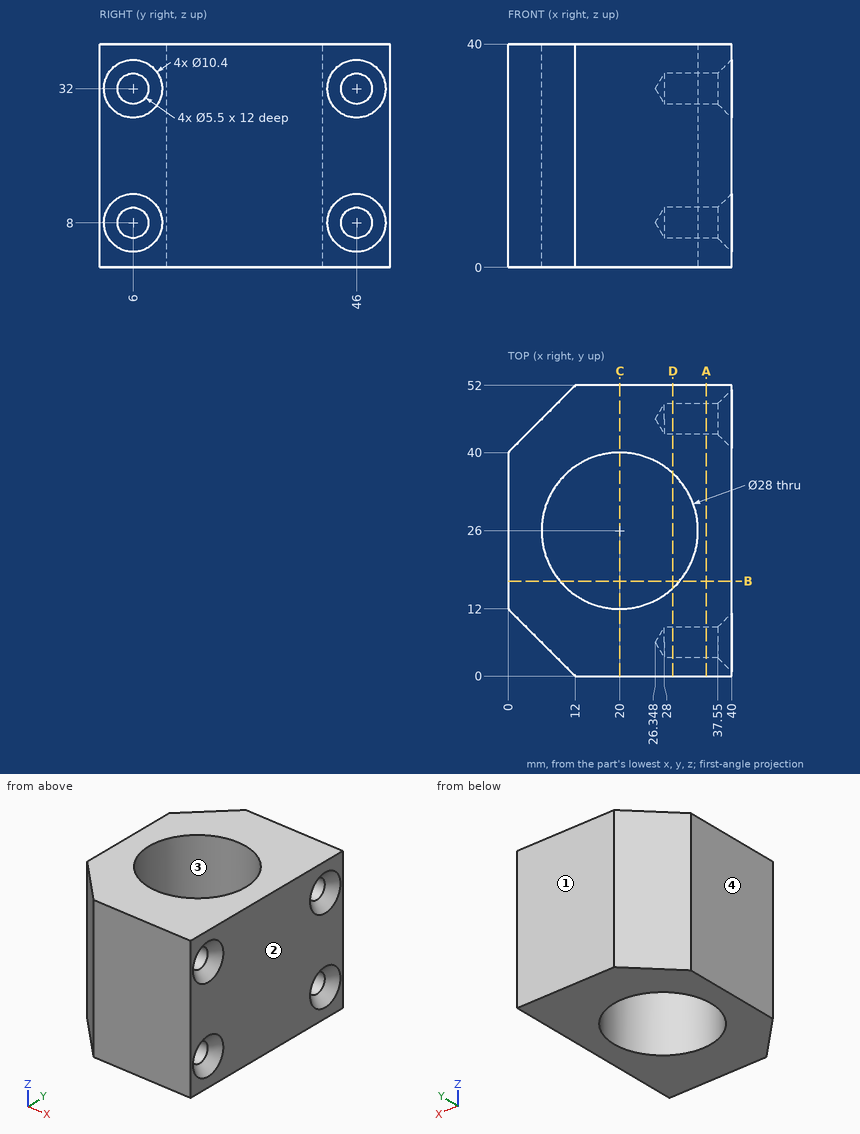
Input: dimensioned drawing with shaded views. Units: mm. Origin: part minimum x, y, z. Give positions to 0.01 mm unless a question says otherwise; leave off trailing zeros. Loops run counter-clockwise (first coordinate to the right, second up) from the corner with the lowest first, then second, coordinate; pieces in that order, holes last. Notation, with made-up numbers: (24, 35.25) -> (82, 35.25) arc R17 ccw to (82, 39.25) -> close; hole circle Ø3 at (-5, -5). An arc over 180 degrees is marked (long way). Use a Markdown table: item, result. Add a question column.
1) Section query D-D, the plane x = 29.5. Return the cut outline in (y, z).
2) Section query B-B, the plane y = 17. Return the cut outline in (x, z), then the cut area to 3 significant figures.
3) Section query A-A, the plane x = 35.5. Return the cut outline in (y, z).
4) Pull-direction query (X, two-part tool) for the marked faces 1, 2, 3 and 4; classes: +X half, -X half, draft (parallel to the pull), parting line (faces both ways), or undercut.
5) Section query C-C, the plane x = 20. Return the cut outline in (y, z).
6) Line query: line 1 along Y through (x, z) = (35.5, 8); line 2 along Z through (x, y) = (32, 6); line 3 along Z through (x, y) = (35.5, 44). Output: solid intervals per line, ascending. Write a range as [from, to].
7) First-contact query: pin 1 (6 mm diameter, centred on x = 8, z = 6, fed in from -Y); pin 2 (7 mm diameter, centred on y = 46, z = 32, fed in from +X); pin 3 (2 mm diameter, centred on x = 7.5, y = 29, fed in from +Z); pin 4 (7 mm diameter, centred on y = 6, z = 8, fed in from -X). Flat tips, straight axial feed; report the tip coordinate or a pass-through.
Numbers:
| question | item | result |
|---|---|---|
| 1 | outline | (0, 0) -> (15.72, 0) -> (15.72, 40) -> (0, 40) -> close; (36.28, 0) -> (52, 0) -> (52, 40) -> (36.28, 40) -> close; hole circle Ø5.5 at (6, 8); hole circle Ø5.5 at (6, 32); hole circle Ø5.5 at (46, 8); hole circle Ø5.5 at (46, 32) |
| 2 | outline | (0, 0) -> (9.28, 0) -> (9.28, 40) -> (0, 40) -> close; (30.72, 0) -> (40, 0) -> (40, 40) -> (30.72, 40) -> close |
| 2 | area | 742 mm2 |
| 3 | outline | (0, 0) -> (52, 0) -> (52, 40) -> (0, 40) -> close; hole circle Ø5.5 at (6, 8); hole circle Ø5.5 at (6, 32); hole circle Ø5.5 at (46, 8); hole circle Ø5.5 at (46, 32) |
| 4 | face 1 | draft |
| 4 | face 2 | +X half |
| 4 | face 3 | undercut |
| 4 | face 4 | -X half |
| 5 | outline | (0, 0) -> (12, 0) -> (12, 40) -> (0, 40) -> close; (40, 0) -> (52, 0) -> (52, 40) -> (40, 40) -> close |
| 6 | line 1 | y = [0, 3.25], [8.75, 43.25], [48.75, 52] |
| 6 | line 2 | z = [0, 5.25], [10.75, 29.25], [34.75, 40] |
| 6 | line 3 | z = [0, 6.11], [9.89, 30.11], [33.89, 40] |
| 7 | pin 1 | stops at y = 1 |
| 7 | pin 2 | stops at x = 38.3 |
| 7 | pin 3 | passes through |
| 7 | pin 4 | stops at x = 2.5 |
